```python
from build123d import *

# Parameters (mm, degrees)
SKETCH1_W           = 60
SKETCH1_H           = 43
BOSS_EXTRUDE1_DEPTH = 5
SKETCH1_3_W         = 10
SKETCH1_3_H         = 43
SKETCH1_3_W_2       = 7
BOSS_EXTRUDE2_DEPTH = 2
SKETCH2_R           = 1.75
CUT_EXTRUDE1_DEPTH  = 2
SKETCH3_R           = 1.75
CUT_EXTRUDE2_DEPTH  = 2
SKETCH4_W           = 3
SKETCH4_H           = 36
BOSS_EXTRUDE3_DEPTH = 9
SKETCH5_W           = 27
SKETCH5_H           = 18
BOSS_EXTRUDE4_DEPTH = 3


with BuildPart() as part:
    # Sketch1 → Boss-Extrude1 (new body)
    with BuildSketch(Plane(origin=(0, 0, 0), x_dir=(1, 0, 0), z_dir=(0, 1, 0))):
        with Locations((-1.5, 0)):
            Rectangle(SKETCH1_W, SKETCH1_H)
    extrude(amount=BOSS_EXTRUDE1_DEPTH)

    # Sketch1_3 → Boss-Extrude2 (add)
    with BuildSketch(Plane(origin=(0, 0, 0), x_dir=(1, 0, 0), z_dir=(0, 1, 0))):
        with Locations((33.5, 0)):
            Rectangle(SKETCH1_3_W, SKETCH1_3_H)
        with Locations((-35, 0)):
            Rectangle(SKETCH1_3_W_2, SKETCH1_3_H)
    extrude(amount=BOSS_EXTRUDE2_DEPTH)

    # Sketch2 → Cut-Extrude1 (cut)
    with BuildSketch(Plane(origin=(0, 2, 0), x_dir=(1, 0, 0), z_dir=(0, 1, 0))):
        with Locations((31.25, 18.25)):
            Circle(SKETCH2_R)
        with Locations((31.25, -18.25)):
            Circle(SKETCH2_R)
    extrude(amount=-CUT_EXTRUDE1_DEPTH, mode=Mode.SUBTRACT)

    # Sketch3 → Cut-Extrude2 (cut)
    with BuildSketch(Plane(origin=(0, 2, 0), x_dir=(1, 0, 0), z_dir=(0, 1, 0))):
        with Locations((-35.25, 18.25)):
            Circle(SKETCH3_R)
        with Locations((-35.25, -18.25)):
            Circle(SKETCH3_R)
    extrude(amount=-CUT_EXTRUDE2_DEPTH, mode=Mode.SUBTRACT)

    # Sketch4 → Boss-Extrude3 (add)
    with BuildSketch(Plane.XZ):
        with Locations((36, 0)):
            Rectangle(SKETCH4_W, SKETCH4_H)
    extrude(amount=BOSS_EXTRUDE3_DEPTH)

    # Sketch5 → Boss-Extrude4 (add)
    with BuildSketch(Plane.XZ):
        with Locations((-9, 11.5)):
            Rectangle(SKETCH5_W, SKETCH5_H)
    extrude(amount=BOSS_EXTRUDE4_DEPTH)


solid = part.part
```
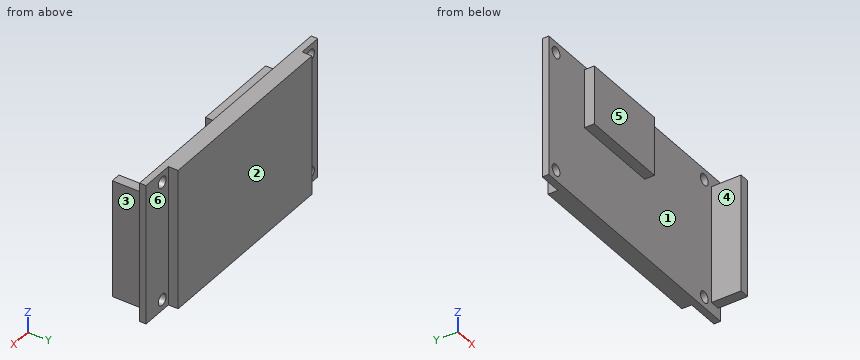
Can you work these out from the model? Positions are in its coordinate system, mm. Face numbers are marked on the shaded views. A direction names the side the tool comes from. Round coordinates to 2 decimals unless told otherwise and drop trailing zeros. Order: outer loops, then holes, each group sorted by start corner. A loop starts at its lowest first (then second) coordinate and runs counter-clockwise, first axis right, second up.
(1) We'd pull the mould along X, two halves only. Please class the marked faces 1, 2 and 3: +X half, -X half, draft (parallel to the pull), parting line (faces both ways), or undercut.
Results are:
face 1: undercut
face 2: draft
face 3: +X half
(2) I'm going to push flat-ended pins straight in: pin 1 (4.5 mm diameter, centred on x = 31.25, z = -18.25, fed in from +Y); pin 2 (3.5 mm diameter, centred on x = 36, y = -4, fed in from -Z); pin 3 (1 mm diameter, centred on y = -5, z = 12, fed in from +X). Where does each tip first touch, or does it pass through?
Results are:
pin 1: stops at y = 2
pin 2: stops at z = -18
pin 3: stops at x = 37.5
(3) On a 3-axis mill with a long thin cutter (end or side, diameter ignored), from which of +Z, -Z, +X, -X, +Y, -Y can I reach the whole of each face in a straight line? I mean the marked faces 4, 5 and 6. Say none if no direction works.
Results are:
face 4: +Z, -Z, -Y
face 5: +Z, -Z, -X, -Y
face 6: +Z, -Z, +X, +Y
(4) If we section it at C-C (z = 11.5): Please give me the cut outline in (x, y), plus the area to 3 significant figures.
Results are:
outline: (-38.5, 0) - (-22.5, 0) - (-22.5, -3) - (4.5, -3) - (4.5, 0) - (34.5, 0) - (34.5, -9) - (37.5, -9) - (37.5, 0) - (38.5, 0) - (38.5, 2) - (28.5, 2) - (28.5, 5) - (-31.5, 5) - (-31.5, 2) - (-38.5, 2) - close
area: 442 mm2
(5) If I drill on L1, parallel to Z at x = 31.25, y = 1.2; L2, parallel to X at y = 0.5, z = -18.25; L3, parallel to X at y = -2.75, z = 17, over which ranges is the centre line in solid material (lowest first)?
Results are:
L1: z = -21.5 to -20, -16.5 to 16.5, 20 to 21.5
L2: x = -38.5 to -37, -33.5 to 29.5, 33 to 38.5
L3: x = -22.5 to 4.5, 34.5 to 37.5
(6) If we section it at B-B (y = -1.75): Please give me the cut outline in (x, z).
Results are:
outline: (-22.5, 2.5) - (4.5, 2.5) - (4.5, 20.5) - (-22.5, 20.5) - close; (34.5, -18) - (37.5, -18) - (37.5, 18) - (34.5, 18) - close
(7) If we section it at D-D (x = -8): Please give me the cut outline in (y, z).
Results are:
outline: (-3, 2.5) - (0, 2.5) - (0, -21.5) - (5, -21.5) - (5, 21.5) - (0, 21.5) - (0, 20.5) - (-3, 20.5) - close
(8) If we section it at A-A (x = -35.25): Please give me the cut outline in (y, z).
Results are:
outline: (0, -21.5) - (2, -21.5) - (2, -20) - (0, -20) - close; (0, -16.5) - (2, -16.5) - (2, 16.5) - (0, 16.5) - close; (0, 20) - (2, 20) - (2, 21.5) - (0, 21.5) - close
